from build123d import *

# Parameters (mm, degrees)
RESSALTO_EXTRUS_O1_DEPTH = 2
ESBO_O2_R                = 1
ESBO_O2_R_2              = 1.5
ESBO_O2_W                = 20
ESBO_O2_H                = 2
CORTE_EXTRUS_O1_DEPTH    = 3


with BuildPart() as part:
    # Esboço1 → Ressalto-extrusão1 (new body)
    with BuildSketch(Plane.XY):
        with BuildLine():
            Line((0, 0), (11, 0))
            Line((11, 0), (59.315981002, 7.73055696))
            ThreePointArc((59.315981002, 7.73055696), (60.521834749, 8.407740649), (61, 9.705438224))
            Line((61, 9.705438224), (61, 18.403988486))
            ThreePointArc((61, 18.403988486), (60.701301617, 19.45545071), (59.894427191, 20.192842868))
            Line((59.894427191, 20.192842868), (33.763932023, 33.258090452))
            ThreePointArc((33.763932023, 33.258090452), (31.746745958, 35.101570847), (31, 37.730226407))
            Line((31, 37.730226407), (31, 49.640056464))
            Line((31, 49.640056464), (33.315981002, 50.010613424))
            ThreePointArc((33.315981002, 50.010613424), (34.521834749, 50.687797112), (35, 51.985494688))
            Line((35, 51.985494688), (35, 63.549919266))
            ThreePointArc((35, 63.549919266), (34.512573863, 64.858399418), (33.287879691, 65.529092145))
            Line((33.287879691, 65.529092145), (7.5, 69.280056464))
            Line((7.5, 69.280056464), (0, 69.280056464))
            Line((0, 69.280056464), (0, 61.780056464))
            Line((0, 61.780056464), (7.5, 61.780056464))
            Line((7.5, 61.780056464), (12.5, 58.780056464))
            Line((12.5, 58.780056464), (12.5, 39.780056464))
            Line((12.5, 39.780056464), (16.346153846, 30.549287233))
            ThreePointArc((16.346153846, 30.549287233), (16.164100589, 28.670656071), (14.5, 27.780056464))
            Line((14.5, 27.780056464), (0, 27.780056464))
            Line((0, 27.780056464), (0, 0))
        make_face()
    ressalto_extrus_o1 = extrude(amount=RESSALTO_EXTRUS_O1_DEPTH)

    # Espelhar1: Ressalto-extrusão1 across plane
    add(ressalto_extrus_o1.mirror(Plane(origin=(0, 0, 0), x_dir=(0, 0, 1), z_dir=(1, 0, 0))))

    # Esboço2 → Corte-extrusão1 (cut, through all)
    with BuildSketch(Plane.XY.offset(2)):
        with Locations((-5, 23.780056464)):
            Circle(ESBO_O2_R)
        with Locations((5, 23.780056464)):
            Circle(ESBO_O2_R)
        with Locations((5, 16.780056464)):
            Circle(ESBO_O2_R)
        with Locations((-5, 16.780056464)):
            Circle(ESBO_O2_R)
        with Locations((0, 20.280056464)):
            Circle(ESBO_O2_R)
        with Locations((-8, 8)):
            Circle(ESBO_O2_R_2)
        with Locations((8, 8)):
            Circle(ESBO_O2_R_2)
        with BuildLine():
            Line((-24, 59.661874645), (-24, 49.661874645))
            ThreePointArc((-24, 49.661874645), (-25.5, 48.161874645), (-27, 49.661874645))
            Line((-27, 49.661874645), (-27, 59.661874645))
            ThreePointArc((-27, 59.661874645), (-25.5, 61.161874645), (-24, 59.661874645))
        make_face()
        with BuildLine():
            Line((24, 59.661874645), (24, 49.661874645))
            ThreePointArc((24, 49.661874645), (25.5, 48.161874645), (27, 49.661874645))
            Line((27, 49.661874645), (27, 59.661874645))
            ThreePointArc((27, 59.661874645), (25.5, 61.161874645), (24, 59.661874645))
        make_face()
        with Locations((-51, 15.407740649)):
            Rectangle(ESBO_O2_W, ESBO_O2_H)
        with Locations((51, 15.407740649)):
            Rectangle(ESBO_O2_W, ESBO_O2_H)
    extrude(amount=-CORTE_EXTRUS_O1_DEPTH, mode=Mode.SUBTRACT)


solid = part.part
Could you check a few things on this model? Use its own coordinates, in mm. A direction names the side the tool comes from. Coordinates: 2 decimals unless noted, no trailing zeros. Order: outer loops, then holes, each group sorted by start corner. A loop starts at its lowest first (then second) coordinate and runs counter-clockwise, first axis right, second up. Notation, with made-up numbers: (-1, 38.5) -> (39, 38.5) arc R10 cw to (39, 55.5) -> close; hole circle Ø8 at (46, 82). An arc over 180 degrees is marked (long way). One line per item, written item: value. Start each with the question number.
1) Imagine slicing it at A-A on y = 57.5. List the corners of the cut face in (x, z) for me.
2) We'd pull the mould along Y, two halves only. Please class faces 4 (the cylindrical face through (-9.2, 7.1, 1)), 5 (the flat face through (1, 27, 2)), 6 (the flat face through (-20.57, 67.38, 0.99)): +Y half, -Y half, draft (parallel to the pull), parting line (faces both ways), or undercut.
3) Imagine slicing it at D-D on z = 0.6. Count the separate pieces of the cut face and the enclosed holes in it, plus the area to 3 significant figures.
4) Which directions (+Z, -Z, +X, -X, +Y, -Y) give clear straight access to the entire face, cutting with the end or side of a thin tool? Please do faces 1 (the cylindrical face through (31.767, 35.069, 0.986)), 2 (the flat face through (-14.396, 35.229, 0.986)), 3 (the cylindrical face through (-31.767, 35.069, 0.986)).
5) I'm going to push flat-ended pins straight in: pin 1 (1 mm diameter, centred on y = 47, z = 1, fed in from -X); pin 2 (1 mm diameter, centred on y = 53.5, z = 1, fed in from -X). Where does each tip first touch, or does it pass through?
6) Imagine slicing it at B-B on x = -25.5. List the corners of the cut face in (y, z) for me.
7) If I drill on L1, parallel to X at y = 57, z = 0.3; L2, parallel to Y at x = 5, z = 0.6; L3, parallel to X at y = 50.5, z = 0.6, over which ranges is the centre line in solid material (lowest first)? Write a range as [from, to].
8) Imagine slicing it at C-C on y = 35.5. List the corners of the cut face in (x, z) for me, plus the area to 3 significant figures.
Answer list:
1. outline: (-35, 0) -> (-27, 0) -> (-27, 2) -> (-35, 2) -> close; (-24, 0) -> (-12.5, 0) -> (-12.5, 2) -> (-24, 2) -> close; (12.5, 0) -> (24, 0) -> (24, 2) -> (12.5, 2) -> close; (27, 0) -> (35, 0) -> (35, 2) -> (27, 2) -> close
2. face 4: undercut
2. face 5: draft
2. face 6: +Y half
3. separate pieces: 1
3. enclosed holes: 10
3. area: 4,490 mm2
4. face 1: +Z, -Z, +X
4. face 2: +Z, -Z
4. face 3: +Z, -Z, -X
5. pin 1: stops at x = -31
5. pin 2: stops at x = -35
6. outline: (2.32, 0) -> (48.16, 0) -> (48.16, 2) -> (2.32, 2) -> close; (61.16, 0) -> (66.66, 0) -> (66.66, 2) -> (61.16, 2) -> close
7. L1: x = [-35, -27], [-24, -12.5], [12.5, 24], [27, 35]
7. L2: y = [0, 15.78], [17.78, 22.78], [24.78, 27.78], [61.78, 69.28]
7. L3: x = [-34.34, -27], [-24, -12.5], [12.5, 24], [27, 34.34]
8. outline: (-31.52, 0) -> (-14.28, 0) -> (-14.28, 2) -> (-31.52, 2) -> close; (14.28, 0) -> (31.52, 0) -> (31.52, 2) -> (14.28, 2) -> close
8. area: 69.0 mm2
